Can you work these out from the model? Positions are in its coordinate system, mm. A direction names the side the tool comes from. Coordinates: 2 decimals unless noted, no trailing zeros. Write each loop counter-clockwise with the first axis right and the second up, starting at its lowest first coordinate (ties: lowest second). Pieces come first, ordered by that corner, then holes.
```python
from build123d import *

# Parameters (mm, degrees)
SCHIZZO1_W                   = 71
SCHIZZO1_H                   = 36
ESTRUSIONE_ESTRUSIONE1_DEPTH = 2
SCHIZZO2_W                   = 66.4
SCHIZZO2_H                   = 31.4
ESTRUSIONE_ESTRUSIONE2_DEPTH = 3
SCHIZZO3_R                   = 5
ESTRUSIONE_ESTRUSIONE3_DEPTH = 5
SCHIZZO4_W                   = 60.4
SCHIZZO4_H                   = 25.4
TAGLIO_ESTRUSIONE1_DEPTH     = 3


with BuildPart() as part:
    # Schizzo1 → Estrusione-Estrusione1 (new body)
    with BuildSketch(Plane(origin=(0, 0, 0), x_dir=(1, 0, 0), z_dir=(0, 1, 0))):
        Rectangle(SCHIZZO1_W, SCHIZZO1_H)
    extrude(amount=ESTRUSIONE_ESTRUSIONE1_DEPTH)

    # Schizzo2 → Estrusione-Estrusione2 (add)
    with BuildSketch(Plane(origin=(0, 2, 0), x_dir=(1, 0, 0), z_dir=(0, 1, 0))):
        Rectangle(SCHIZZO2_W, SCHIZZO2_H)
    extrude(amount=ESTRUSIONE_ESTRUSIONE2_DEPTH)

    # Schizzo3 → Estrusione-Estrusione3 (add)
    with BuildSketch(Plane.XZ):
        with Locations(Location((0, 0, 0), (0, 0, 270))):
            Circle(SCHIZZO3_R)
    extrude(amount=ESTRUSIONE_ESTRUSIONE3_DEPTH)

    # Schizzo4 → Taglio-Estrusione1 (cut)
    with BuildSketch(Plane(origin=(0, 5, 0), x_dir=(1, 0, 0), z_dir=(0, 1, 0))):
        Rectangle(SCHIZZO4_W, SCHIZZO4_H)
    extrude(amount=-TAGLIO_ESTRUSIONE1_DEPTH, mode=Mode.SUBTRACT)


solid = part.part
```
1. We'd pull the mould along Z, two halves only. Please class faces 1 (the face through (-30.2, 4, 0)), 2 (the face through (-33.2, 3, 0)), 3 (the face through (0, 3, 15.7)): released by +Z, released by -Z, zero draft, split by the parting line, or undercut.
2. If we section it at C-C, the plane y = -1.75: List the corners of the cut face in (x, z) for me.
3. If we section it at D-D, the plane x = 0: List the corners of the cut face in (y, z) for me, plus the area to 3 significant figures.
4. If we section it at B-B, the plane x = -9.5: List the corners of the cut face in (y, z) for me, plus the area to 3 significant figures.
5. I'm going to push flat-ended pins straight in: P1, Ø3.5, axis at x = 9, y = 4, coming from the -Z side; P2, Ø3.5, axis at y = 4, z = -7, coming from the +X side; P3, Ø6, axis at x = -21.5, y = -4, coming from the +Z side; P4, Ø12, axis at x = -20.5, z = -2, coming from the -Y side. Where does each tip first touch, or does it pass through?
6. If we section it at A-A, the plane z = 0: List the corners of the cut face in (x, y) for me, plus the area to 3 significant figures.
7. If I drill on L1, parallel to Z at x = 22, y = 4.25; L2, parallel to X at y = 3.5, z = 7.5; L3, parallel to Y at x = -17.5, z = -4.5, over which ranges is the centre line in solid material (lowest first)?
8. Which directions (+Z, -Z, +X, -X, +Y, -Y) give clear straight access to the entire face, cutting with the end or side of a thin tool? Please do faces 4 (the face through (0, 1, -18)), 5 (the face through (33.2, 3, 0)), 6 (the face through (0, 3, -15.7)), 7 (the face through (-4.88, -2.46, 1.08)), 8 (the face through (30.2, 4, 0)).
Answers:
1. face 1: undercut
1. face 2: zero draft
1. face 3: released by +Z
2. outline: circle Ø10 at (0, 0)
3. outline: (-5, -5) - (0, -5) - (0, -18) - (2, -18) - (2, -15.7) - (5, -15.7) - (5, -12.7) - (2, -12.7) - (2, 12.7) - (5, 12.7) - (5, 15.7) - (2, 15.7) - (2, 18) - (0, 18) - (0, 5) - (-5, 5) - close
3. area: 140 mm2
4. outline: (0, -18) - (2, -18) - (2, -15.7) - (5, -15.7) - (5, -12.7) - (2, -12.7) - (2, 12.7) - (5, 12.7) - (5, 15.7) - (2, 15.7) - (2, 18) - (0, 18) - close
4. area: 90.0 mm2
5. P1: stops at z = -15.7
5. P2: stops at x = 33.2
5. P3: passes through
5. P4: stops at y = 0
6. outline: (-35.5, 0) - (-5, 0) - (-5, -5) - (5, -5) - (5, 0) - (35.5, 0) - (35.5, 2) - (33.2, 2) - (33.2, 5) - (30.2, 5) - (30.2, 2) - (-30.2, 2) - (-30.2, 5) - (-33.2, 5) - (-33.2, 2) - (-35.5, 2) - close
6. area: 210 mm2
7. L1: z = -15.7 to -12.7, 12.7 to 15.7
7. L2: x = -33.2 to -30.2, 30.2 to 33.2
7. L3: y = 0 to 2
8. face 4: -Z, +X, -X, +Y, -Y
8. face 5: +Z, -Z, +X, +Y
8. face 6: -Z, +X, -X, +Y
8. face 7: -Y
8. face 8: +Y
